For this review, take the finished solid that the model builds, in its own axes (mm). Give positions to 0.01 mm unless a question says otherwise; leave off trailing zeros. Loops run counter-clockwise (first coordinate to the right, second up) from the corner with the lowest first, then second, coordinate; pieces in that order, holes last.
```python
from build123d import *

# Parameters (mm, degrees)
SKETCH2_R           = 4
BOSS_EXTRUDE1_DEPTH = 3


with BuildPart() as part:
    # Sketch2 → Boss-Extrude1 (new body)
    # profile 1 of 3: a face of its own
    with BuildSketch(Plane.XY.offset(29.670544835)):
        with BuildLine():
            ThreePointArc((6.802372388, 14.495325214), (-28.853343247, 37.601496731), (-65.190306526, 15.582179772))
            Line((-65.190306526, 15.582179772), (-50.268412727, 15.582179772))
            ThreePointArc((-50.268412727, 15.582179772), (-28.754344017, 25.097072211), (-7.754551371, 14.495325214))
            Line((-7.754551371, 14.495325214), (6.802372388, 14.495325214))
        make_face()
        with Locations((-54.457143935, 20.606054181)):
            Circle(SKETCH2_R, mode=Mode.SUBTRACT)
        with Locations((-30.871357497, 31.547179678)):
            Circle(SKETCH2_R, mode=Mode.SUBTRACT)
        with Locations((-6.457143935, 22.606054181)):
            Circle(SKETCH2_R, mode=Mode.SUBTRACT)
    # profile 2 of 3: a face of its own
    with BuildSketch(Plane.XY.offset(29.670544835)):
        with BuildLine():
            ThreePointArc((-67.915477314, 25.484479418), (-69.818945991, 22.649515101), (-71.513826382, 19.685127113))
            Line((-71.513826382, 19.685127113), (-71.513826382, 15.582179772))
            Line((-71.513826382, 15.582179772), (-65.190306526, 15.582179772))
            ThreePointArc((-65.190306526, 15.582179772), (-28.853343247, 37.601496731), (6.802372388, 14.495325214))
            Line((6.802372388, 14.495325214), (14.938830252, 14.495325214))
            ThreePointArc((14.938830252, 14.495325214), (14.389447504, 15.874234692), (13.797248858, 17.235305417))
            ThreePointArc((13.797248858, 17.235305417), (8.501873451, 18.851359524), (9.893531234, 24.21008327))
            ThreePointArc((9.893531234, 24.21008327), (6.804255556, 28.287659534), (3.294383766, 32.009359739))
            ThreePointArc((3.294383766, 32.009359739), (-2.22078734, 31.524056472), (-2.93787796, 37.013902793))
            ThreePointArc((-2.93787796, 37.013902793), (-7.329691445, 39.637302632), (-11.978161336, 41.773181859))
            ThreePointArc((-11.978161336, 41.773181859), (-16.909941136, 39.257197046), (-19.63134861, 44.078667044))
            ThreePointArc((-19.63134861, 44.078667044), (-24.686110043, 44.86583873), (-29.796210715, 45.104843995))
            ThreePointArc((-29.796210715, 45.104843995), (-29.792572401, 45.00640165), (-29.791359384, 44.907899562))
            ThreePointArc((-29.791359384, 44.907899562), (-33.524574673, 40.916806239), (-37.755772343, 44.375518221))
            ThreePointArc((-37.755772343, 44.375518221), (-42.737345236, 43.211824139), (-47.564881022, 41.519148556))
            ThreePointArc((-47.564881022, 41.519148556), (-47.288818763, 40.699632679), (-47.195341682, 39.839935825))
            ThreePointArc((-47.195341682, 39.839935825), (-50.171922049, 35.97307505), (-54.67164781, 37.861225208))
            ThreePointArc((-54.67164781, 37.861225208), (-58.85455429, 34.916136792), (-62.696480095, 31.538288585))
            ThreePointArc((-62.696480095, 31.538288585), (-61.762829246, 30.210656667), (-61.433540443, 28.621355152))
            ThreePointArc((-61.433540443, 28.621355152), (-63.691092092, 25.020817172), (-67.915477314, 25.484479418))
        make_face()
    # profile 3 of 3: a face of its own
    with BuildSketch(Plane.XY.offset(29.670544835)):
        with BuildLine():
            ThreePointArc((22.885501432, 14.495325214), (-18.849868318, 51.573504594), (-71.513826382, 33.049466285))
            Line((-71.513826382, 33.049466285), (-71.513826382, 19.685127113))
            ThreePointArc((-71.513826382, 19.685127113), (-69.818945991, 22.649515101), (-67.915477314, 25.484479418))
            ThreePointArc((-67.915477314, 25.484479418), (-68.463131728, 31.233169971), (-62.696480095, 31.538288585))
            ThreePointArc((-62.696480095, 31.538288585), (-58.85455429, 34.916136792), (-54.67164781, 37.861225208))
            ThreePointArc((-54.67164781, 37.861225208), (-53.025926756, 43.396473227), (-47.564881022, 41.519148556))
            ThreePointArc((-47.564881022, 41.519148556), (-42.737345236, 43.211824139), (-37.755772343, 44.375518221))
            ThreePointArc((-37.755772343, 44.375518221), (-34.156345949, 48.891212858), (-29.796210715, 45.104843995))
            ThreePointArc((-29.796210715, 45.104843995), (-24.686110043, 44.86583873), (-19.63134861, 44.078667044))
            ThreePointArc((-19.63134861, 44.078667044), (-15.256521979, 47.055857815), (-11.756175362, 43.087187195))
            ThreePointArc((-11.756175362, 43.087187195), (-11.812062273, 42.420874994), (-11.978161336, 41.773181859))
            ThreePointArc((-11.978161336, 41.773181859), (-7.329691445, 39.637302632), (-2.93787796, 37.013902793))
            ThreePointArc((-2.93787796, 37.013902793), (1.531436617, 38.443369839), (4.283705221, 34.642953235))
            ThreePointArc((4.283705221, 34.642953235), (4.028215481, 33.23631081), (3.294383766, 32.009359739))
            ThreePointArc((3.294383766, 32.009359739), (6.804255556, 28.287659534), (9.893531234, 24.21008327))
            ThreePointArc((9.893531234, 24.21008327), (13.942318539, 24.297464692), (15.992357809, 20.804950819))
            ThreePointArc((15.992357809, 20.804950819), (15.399670841, 18.709666137), (13.797248858, 17.235305417))
            ThreePointArc((13.797248858, 17.235305417), (14.389447504, 15.874234692), (14.938830252, 14.495325214))
            Line((14.938830252, 14.495325214), (22.885501432, 14.495325214))
        make_face()
    extrude(amount=BOSS_EXTRUDE1_DEPTH)


solid = part.part
```
Item 1: The part is to be moulded in two halves that separate along Y. For faces 1 (the cylindrical face through (-4.31, 25.98, 31.15)), 2 (the flat face through (-61, 15.582, 31)), 3 (the flat face through (-71.514, 24, 31)), 4 (the cylindrical face through (-27.176, 30.015, 31.15)), say which applies: released by +Y, released by -Y, zero draft, split by the parting line, or undercut.
Answer:
face 1: undercut
face 2: released by -Y
face 3: zero draft
face 4: undercut
Item 2: For L1, parallel to X at y = 33, z = 32.15; L2, parallel to Y at x = -33.5, z = 31.1; L3, parallel to X at y = 46, z = 32.55, list the stretches that pass through material, from the lowest coordinate up.
Answer:
L1: x = -71.51 to -34.6, -27.14 to -3.36, 3.93 to 12.64
L2: y = 24.81 to 28.53, 34.56 to 40.92, 48.9 to 52.46
L3: x = -55.59 to -37.64, -29.94 to -18.5, -13.01 to -3.32
Item 3: Take a section at D-D on x = -24. Give the boundary of the cut face in (y, z), and give its area (3 significant figures).
Answer:
outline: (24.56, 29.67) - (52.33, 29.67) - (52.33, 32.67) - (24.56, 32.67) - close
area: 83.3 mm2
Item 4: Take a section at B-B on z = 30.5. State how many separate pieces and enclosed holes the cut face has, and give its area (3 significant figures).
Answer:
separate pieces: 1
enclosed holes: 9
area: 2,020 mm2
Item 5: Take a section at A-A on x = -36.5. Give the boundary of the cut face in (y, z), and give its area (3 significant figures).
Answer:
outline: (24.19, 29.67) - (41.96, 29.67) - (41.96, 32.67) - (24.19, 32.67) - close; (47.85, 29.67) - (52.15, 29.67) - (52.15, 32.67) - (47.85, 32.67) - close
area: 66.2 mm2
Item 6: Take a section at C-C on x = -65. Give the boundary of the cut face in (y, z), and give its area (3 significant figures).
Answer:
outline: (15.58, 29.67) - (24.64, 29.67) - (24.64, 32.67) - (15.58, 32.67) - close; (32.6, 29.67) - (39.58, 29.67) - (39.58, 32.67) - (32.6, 32.67) - close
area: 48.1 mm2
Item 7: Clearance check with flat-ended pins moving along their axes: pin 1 Ø13 at (x, y) = (-54.46, 20.61) entering from -Z; pin 2 Ø5 at (x, y) = (-30.87, 31.55) entering from -Z; pin 3 Ø0.9 at (x, z) = (-58.5, 30.5) entering from -Y. State where each tip first meets the part, or that it passes through.
Answer:
pin 1: stops at z = 29.67
pin 2: passes through
pin 3: stops at y = 15.58
